```python
from build123d import *

# Parameters (mm, degrees)
F0_W     = 457.2
F0_H     = 1219.2
F1_DEPTH = 6.35
F2_SIZE  = 6.34999
F3_SIZE  = 6.34999


# Not quite as in the source:
# - a fillet or chamfer is up to 0.001 mm smaller than in the source, because OpenCascade refuses the exact size


with BuildPart() as f1:
    # F0 (on Front) → F1 (new body)
    with BuildSketch(Plane.XZ):
        Rectangle(F0_W, F0_H)
    extrude(amount=F1_DEPTH)

    # F2 (size 6.35 in the source; OpenCascade refuses exactly that, so slightly less here)
    f2_edges = [f1.edges().sort_by_distance(p)[0] for p in [
        (-228.6, 0, 0),
    ]]
    chamfer(f2_edges, length=F2_SIZE)

    # F3 (size 6.35 in the source; OpenCascade refuses exactly that, so slightly less here)
    f3_edges = [f1.edges().sort_by_distance(p)[0] for p in [
        (228.6, 0, 0),
    ]]
    chamfer(f3_edges, length=F3_SIZE)


solid = f1.part
```
Input: part model. Units: mm. Frame: model coordinates. Coordinates: 2 decimals unless noted, no trailing zeros. Loops run counter-clockwise (first coordinate to the right, second up) from the corner with the lowest first, then second, coordinate; pieces in that order, holes last. Notation, with made-up numbers: M 39.5,28.25 L 94.5,28.25 A8 cw 94.5,42.25 Z; hole C 85.5,84.25 d6. An arc over 180 degrees is marked long. Answer in a Markdown table with one row per item.
1. Section A-A, the plane y = -2.25. Output: boundary loops of the cut face in (x, z).
Response:
| item | result |
|---|---|
| outline | M -224.5,-609.6 L 224.5,-609.6 L 224.5,609.6 L -224.5,609.6 Z |
2. First-contact query: pin 1 (2 mm diameter, centred on y = -2, z = -163, fed in from -X); pin 2 (1.5 mm diameter, centred on y = -5, z = 10, fed in from -X). Flat tips, straight axial feed; report the tip coordinate or a pass-through.
Response:
| item | result |
|---|---|
| pin 1 | stops at x = -225.25 |
| pin 2 | stops at x = -228 |
3. Material intervals for line 1 (X direction, y = -0.25, z = 240.5); line 2 (X direction, y = -3.5, z = 470), sorted ascending.
Response:
| item | result |
|---|---|
| line 1 | x = -222.5 to 222.5 |
| line 2 | x = -225.75 to 225.75 |
